Could you check a few things on this model? Use its own coordinates, in mm. A direction names the side the tool comes from. Give positions to 0.01 mm unless a question says otherwise; leave off trailing zeros. Order: outer loops, then holes, each group sorted by start corner. A loop starts at its lowest first (then second) coordinate and runs counter-clockwise, first axis right, second up. Notation, with made-up numbers: M 62,22.5 L 91,22.5 A27 cw 91,41.5 Z; hole C 34,89.25 d11. An arc over 180 degrees is marked long. Answer in a Markdown table with one row per item. Add a question column.
```python
from build123d import *

# Parameters (mm, degrees)
SKETCH_1_R      = 2.5
EXTRUDE_1_DEPTH = 3.6
EXTRUDE_START   = -4.9
SKETCH_2_R      = 3.1
SKETCH_2_R_2    = 2.5
EXTRUDE_2_DEPTH = 4.9
FILLET_1_R      = 0.5


with BuildPart() as part:
    # 草图1 → 凸台-拉伸1 (new body)
    with BuildSketch(Plane(origin=(0, 0, 0), x_dir=(1, 0, 0), z_dir=(0, 1, 0))):
        Polygon((4, 0), (2, 3.464101615), (-2, 3.464101615), (-4, 0), (-2, -3.464101615), (2, -3.464101615), align=None)
        with Locations(Location((0, 0, 0), (0, 0, 270))):
            Circle(SKETCH_1_R, mode=Mode.SUBTRACT)
    extrude(amount=EXTRUDE_1_DEPTH)

    # 草图4 → 切除-旋转1 (revolve, cut)
    with BuildSketch(Plane(origin=(0, 0, 0), x_dir=(-0.49999999999999806, 0, 0.8660254037844398), z_dir=(-0.8660254037844397, 0, -0.499999999999998))):
        Polygon((0, 5.609401077), (-4, 3.3), (-4, 5.663718026), (-4, 6.109401077), (0, 6.109401077), align=None)
        Polygon((0, -2.509401077), (0, -2.009401077), (-4, 0.3), (-4, -2.063718026), (-4, -2.509401077), align=None)
    revolve(axis=Axis((0, 6.109401077, 0), (0, 1, 0)), mode=Mode.SUBTRACT)

    # 草图2 → 凸台-拉伸2 (add)
    with BuildSketch(Plane(origin=(0, 3.6, 0), x_dir=(1, 0, 0), z_dir=(0, 1, 0)).offset(EXTRUDE_START)):
        with Locations(Location((0, 0, 0), (0, 0, 270))):
            Circle(SKETCH_2_R)
        with Locations(Location((0, 0, 0), (0, 0, 270))):
            Circle(SKETCH_2_R_2, mode=Mode.SUBTRACT)
    extrude(amount=EXTRUDE_2_DEPTH)

    # 圆角1
    fillet_1_edges = [part.edges().sort_by_distance(p)[0] for p in [
        (0, -1.3, -3.1),
    ]]
    fillet(fillet_1_edges, radius=FILLET_1_R)


solid = part.part
```
1. Thinking about a two-plate mould opening in X: for faces 3 (the conical face through (3.664, 3.494, 0.007)), 4 (the cylindrical face through (-2.44, 1.12, -0.54)), 5 (the flat face through (2.3, 3.6, 1.5)), which applies, pulls with the +X half, pulls with the -X half, needs draft (parallel to the pull), parting line crosses it, or undercut?
2. Suppose I cut it at B-B on x = 0. List the corners of the cut face in (y, z) for me, plus the area to 3 significant figures.
3. For faces 1 (the cylindrical face through (0.931, -0.406, 2.957)), 2 (the conical face through (1.83, 3.49, 3.18)), which set-ups out of +Z, -Z, +X, -X, +Y, -Y let a thin tool reach every point of the face, with its end or its side?
4. Will these pins go through, and if not, where does the flat tip stop? P1, Ø1.5, axis at y = 1.5, z = 2, coming from the +X side; P2, Ø1, axis at x = -2.5, y = 0, coming from the -Z side.
5. Suppose I cut it at C-C on y = -0.5. List the corners of the cut face in (x, z) for me, plus the area to 3 significant figures.
6. Suppose I cut it at A-A on y = 3.2. List the corners of the cut face in (x, z) for me, plus the area to 3 significant figures.
7. If I drill on line 1 along Z through (x, y) = (1.5, 0.5); line 2 along Z through (x, y) = (1.25, -0.25); line 3 along Y through (x, z) = (2.75, 1.5), over which ranges is the centre line in solid material (lowest first)? Write a range as [from, to].
Findings below:
| question | item | result |
|---|---|---|
| 1 | face 3 | pulls with the +X half |
| 1 | face 4 | undercut |
| 1 | face 5 | needs draft |
| 2 | outline | M -1.3,-2.6 A0.5 ccw -0.8,-3.1 L 0,-3.1 L 0,-3.46 L 3.6,-3.46 L 3.6,-2.5 L -1.3,-2.5 Z; M -1.3,2.5 L 3.6,2.5 L 3.6,3.46 L 0,3.46 L 0,3.1 L -0.8,3.1 A0.5 ccw -1.3,2.6 Z |
| 2 | area | 8.39 mm2 |
| 3 | face 1 | -Y |
| 3 | face 2 | +Z, +X, +Y |
| 4 | P1 | x = 3.28 |
| 4 | P2 | z = -3.34 |
| 5 | outline | C 0,0 d6.2; hole C 0,0 d5 |
| 5 | area | 10.6 mm2 |
| 6 | outline | M -4,0 L -2,-3.46 L 2,-3.46 L 4,0 L 2,3.46 L -2,3.46 Z; hole C 0,0 d5 |
| 6 | area | 21.9 mm2 |
| 7 | line 1 | [-3.46, -2], [2, 3.46] |
| 7 | line 2 | [-2.84, -2.17], [2.17, 2.84] |
| 7 | line 3 | [0, 3.6] |
